Input: part model. Units: mm. Frame: model coordinates. A direction names the side the tool comes from. Coordinates: 2 decimals unless noted, no trailing zeros. Write each loop counter-clockwise with the first axis right and the second up, starting at its lowest first coordinate (ties: lowest second). Pieces come first, ordered by that corner, then holes. Notation, with made-up numbers: (44, 36.25) - (102, 36.25) arc R16 cw to (102, 65.25) - close; hole circle Ø2 at (49, -29). An arc over 180 degrees is marked (long way). Put each result on its own line as item: value. Start each with the question number.
1. Cut plane B-B, the plane z = 2.75. Return loops of the section in (x, y), and give its area (3 significant figures).
2. Pull-direction query (Z, two-part tool) for faces 5 (the cylindrical face through (3.925, 2.299, 5.886)), 6 (the flat face through (13.5, 10.5, 0)), 7 (the flat face through (2.2, 1.4, 5.2)), 8 (the flat face through (21.75, 2.91, 2.96)); classes: released by +Z, released by -Z, zero draft, split by the parting line, or undercut.
3. Access query for faces 1 (the flat face through (21.5, 6, 3)), 2 (the flat face through (24.8, 1.4, 5.2)), 3 (the flat face through (19, 9, 0.75)), 4 (the flat face through (18.5, 9, 5.6)). Directions: +Z, -Z, +X, -X, +Y, -Y. A direction counts if a zero-diameter tool reaches every point of the face in a straight line with its end or side. Return the directions, or none.
4. Cut plane D-D, the plane z = 1.25. Return loops of the section in (x, y), and give its area (3 significant figures).
5. Cut plane A-A, the plane y = 8.75. Return loops of the section in (x, z).
6. Line query: line 1 (X direction, y = 0.6, z = 3); line 2 (X direction, y = 5.5, z = 4); line 3 (Y direction, x = 23, z = 1.75). Output: solid intervals per line, ascending.
7. Cut plane C-C, the plane y = 5.5. Return loops of the section in (x, z).
8. Pin query (flat end, axial travel): pin 1 (0.5 mm diameter, centred on x = 24.5, y = 1.5, fed in from +Z); pin 2 (1 mm diameter, centred on y = 9, z = 1, fed in from +X); pin 3 (1.3 mm diameter, centred on x = 25, z = 4, fed in from +Y). Return the tip coordinate at first contact, or that it passes through.
from build123d import *

# Parameters (mm, degrees)
AUFSATZ_LINEAR_AUSTRAGEN1_DEPTH = 6
SKIZZE4_R                       = 1
SCHNITT_LINEAR_AUSTRAGEN1_DEPTH = 3
SCHNITT_LINEAR_AUSTRAGEN2_DEPTH = 2
VERRUNDUNG1_R                   = 0.4
SCHNITT_LINEAR_AUSTRAGEN4_DEPTH = 3
AUFSATZ_LINEAR_AUSTRAGEN2_DEPTH = 0.75
SCHNITT_LINEAR_AUSTRAGEN5_DEPTH = 6


with BuildPart() as part:
    # Skizze1 → Aufsatz-Linear austragen1 (new body)
    with BuildSketch(Plane.XY):
        Polygon((0, 0), (7.5, 0), (7.5, 10), (19.5, 10), (19.5, 0), (27, 0), (27, 1), (21.5, 3), (21.5, 12), (5.5, 12), (5.5, 3), (0, 1), align=None)
    extrude(amount=AUFSATZ_LINEAR_AUSTRAGEN1_DEPTH)

    # Skizze4 → Schnitt-Linear austragen1 (cut)
    with BuildSketch(Plane.XZ):
        with Locations(Location((24.25, 3, 0), (0, 0, 270))):
            Circle(SKIZZE4_R)
    schnitt_linear_austragen1 = extrude(amount=-SCHNITT_LINEAR_AUSTRAGEN1_DEPTH, mode=Mode.SUBTRACT)

    # Skizze5 → Schnitt-Linear austragen2 (cut)
    with BuildSketch(Plane(origin=(0, 3, 0), x_dir=(-1, 0, 0), z_dir=(0, -1, 0))):
        with BuildLine():
            Line((-24.25, -5.2), (-27, -5.2))
            Line((-27, -5.2), (-27, -0.8))
            Line((-27, -0.8), (-24.25, -0.8))
            ThreePointArc((-24.25, -0.8), (-22.05, -3), (-24.25, -5.2))
        make_face()
    schnitt_linear_austragen2 = extrude(amount=SCHNITT_LINEAR_AUSTRAGEN2_DEPTH, mode=Mode.SUBTRACT)

    # Spiegeln1: Schnitt-Linear austragen1, Schnitt-Linear austragen2 across plane
    add(schnitt_linear_austragen1.mirror(Plane(origin=(13.5, 0, 0), x_dir=(0, 0, 1), z_dir=(1, 0, 0))), mode=Mode.SUBTRACT)
    add(schnitt_linear_austragen2.mirror(Plane(origin=(13.5, 0, 0), x_dir=(0, 0, 1), z_dir=(1, 0, 0))), mode=Mode.SUBTRACT)

    # Verrundung1
    verrundung1_edges = [part.edges().sort_by_distance(p)[0] for p in [
        (2.75, 2, 0),
        (5.5, 7.5, 0),
        (21.5, 7.5, 0),
        (24.25, 2, 0),
        (24.25, 2, 6),
        (21.5, 7.5, 6),
        (5.5, 7.5, 6),
        (2.75, 2, 6),
    ]]
    fillet(verrundung1_edges, radius=VERRUNDUNG1_R)

    # Skizze7 → Schnitt-Linear austragen4 (cut)
    with BuildSketch(Plane(origin=(0, 3, 0), x_dir=(-1, 0, 0), z_dir=(0, -1, 0))):
        with BuildLine():
            Line((-24.05, -6), (-27.346568129, -6))
            Line((-27.346568129, -6), (-27.346568129, 0))
            Line((-27.346568129, 0), (-23.943800363, 0))
            ThreePointArc((-23.943800363, 0), (-26.341645128, -2.958498156), (-24.05, -6))
        make_face()
    schnitt_linear_austragen4 = extrude(amount=SCHNITT_LINEAR_AUSTRAGEN4_DEPTH, mode=Mode.SUBTRACT)

    # Spiegeln2: Schnitt-Linear austragen4 across plane
    add(schnitt_linear_austragen4.mirror(Plane(origin=(13.5, 0, 0), x_dir=(0, 0, 1), z_dir=(1, 0, 0))), mode=Mode.SUBTRACT)

    # Skizze8 → Aufsatz-Linear austragen2 (add)
    with BuildSketch(Plane.XY.offset(6)):
        Polygon((9.5, 10), (7.5, 8), (7.5, 10), align=None)
        Polygon((17.5, 10), (19.5, 10), (19.5, 8), align=None)
    aufsatz_linear_austragen2 = extrude(amount=-AUFSATZ_LINEAR_AUSTRAGEN2_DEPTH)

    # Spiegeln3: Aufsatz-Linear austragen2 across plane
    add(aufsatz_linear_austragen2.mirror(Plane.XY.offset(3)))

    # Skizze9 → Schnitt-Linear austragen5 (cut)
    with BuildSketch(Plane.XY.offset(6)):
        Polygon((5.5, 12), (5.5, 10), (7.5, 12), align=None)
    schnitt_linear_austragen5 = extrude(amount=-SCHNITT_LINEAR_AUSTRAGEN5_DEPTH, mode=Mode.SUBTRACT)

    # Spiegeln4: Schnitt-Linear austragen5 across plane
    add(schnitt_linear_austragen5.mirror(Plane(origin=(13.5, 0, 0), x_dir=(0, 0, 1), z_dir=(1, 0, 0))), mode=Mode.SUBTRACT)


solid = part.part
Report:
1. outline: (0.67, 0) - (1.78, 0) - (1.78, 1) - (0.67, 1) - close; (3.72, 0) - (7.5, 0) - (7.5, 10) - (19.5, 10) - (19.5, 0) - (23.28, 0) - (23.28, 1) - (22.06, 1) - (22.06, 2.79) - (21.5, 3) - (21.5, 10) - (19.5, 12) - (7.5, 12) - (5.5, 10) - (5.5, 3) - (4.94, 2.79) - (4.94, 1) - (3.72, 1) - close; (25.22, 0) - (26.33, 0) - (26.33, 1) - (25.22, 1) - close
1. area: 75.9 mm^2
2. face 5: released by +Z
2. face 6: released by -Z
2. face 7: undercut
2. face 8: zero draft
3. face 1: +Z, -Z, +X, +Y
3. face 2: +X, +Y
3. face 3: -Y
3. face 4: +Z, -Z, -Y
4. outline: (1.21, 0) - (7.5, 0) - (7.5, 10) - (19.5, 10) - (19.5, 0) - (25.79, 0) - (25.79, 1) - (22.92, 1) - (22.92, 2.48) - (21.5, 3) - (21.5, 10) - (19.5, 12) - (7.5, 12) - (5.5, 10) - (5.5, 3) - (4.08, 2.48) - (4.08, 1) - (1.21, 1) - close
4. area: 81.5 mm^2
5. outline: (5.5, 0.4) arc R0.4 ccw to (5.9, 0) - (8.25, 0) - (8.25, 0.75) - (7.5, 0.75) - (7.5, 5.25) - (8.25, 5.25) - (8.25, 6) - (5.9, 6) arc R0.4 ccw to (5.5, 5.6) - close; (18.75, 0) - (21.1, 0) arc R0.4 ccw to (21.5, 0.4) - (21.5, 5.6) arc R0.4 ccw to (21.1, 6) - (18.75, 6) - (18.75, 5.25) - (19.5, 5.25) - (19.5, 0.75) - (18.75, 0.75) - close
6. line 1: x = 0.66 to 1.75, 3.75 to 7.5, 19.5 to 23.25, 25.25 to 26.34
6. line 2: x = 5.5 to 7.5, 19.5 to 21.5
6. line 3: y = 0 to 1
7. outline: (5.5, 0.4) arc R0.4 ccw to (5.9, 0) - (7.5, 0) - (7.5, 6) - (5.9, 6) arc R0.4 ccw to (5.5, 5.6) - close; (19.5, 0) - (21.1, 0) arc R0.4 ccw to (21.5, 0.4) - (21.5, 5.6) arc R0.4 ccw to (21.1, 6) - (19.5, 6) - close
8. pin 1: stops at z = 5.94
8. pin 2: stops at x = 21.5
8. pin 3: stops at y = 1
